```python
from build123d import *

# Parameters (mm, degrees)
SKETCH1_W            = 63
SKETCH1_H            = 76
BOSS_EXTRUDE1_DEPTH  = 1.5
SKETCH2_W            = 9
SKETCH2_H            = 74
BOSS_EXTRUDE2_DEPTH  = 11.5
SKETCH3_W            = 7
SKETCH3_H            = 8
BOSS_EXTRUDE3_DEPTH  = 3.5
SKETCH4_W            = 11
SKETCH4_H            = 2
BOSS_EXTRUDE4_DEPTH  = 3
SKETCH5_R            = 0.325
BOSS_EXTRUDE5_DEPTH  = 6
SKETCH6_W            = 6
SKETCH6_H            = 2
BOSS_EXTRUDE6_DEPTH  = 2.5
SKETCH8_W            = 7.2
SKETCH8_H            = 5.5
BOSS_EXTRUDE8_DEPTH  = 4.2
SKETCH9_W            = 5.5
SKETCH9_H            = 6.1
BOSS_EXTRUDE9_DEPTH  = 2
SKETCH10_R           = 1.5
BOSS_EXTRUDE10_DEPTH = 1.7
SKETCH11_W           = 5.5
SKETCH11_H           = 6.1
BOSS_EXTRUDE11_DEPTH = 2
SKETCH12_R           = 1.5
BOSS_EXTRUDE12_DEPTH = 1.7


with BuildPart() as part:
    # Sketch1 → Boss-Extrude1 (new body)
    with BuildSketch(Plane(origin=(0, 0, 0), x_dir=(1, 0, 0), z_dir=(0, 1, 0))):
        with Locations((31.5, 38)):
            Rectangle(SKETCH1_W, SKETCH1_H)
    extrude(amount=BOSS_EXTRUDE1_DEPTH)

    # Sketch2 → Boss-Extrude2 (add)
    with BuildSketch(Plane(origin=(0, 1.5, 0), x_dir=(1, 0, 0), z_dir=(0, 1, 0))):
        with Locations((7, 38)):
            Rectangle(SKETCH2_W, SKETCH2_H)
    extrude(amount=BOSS_EXTRUDE2_DEPTH)

    # Sketch3 → Boss-Extrude3 (add)
    with BuildSketch(Plane.XZ):
        with Locations((12.5, -19)):
            Rectangle(SKETCH3_W, SKETCH3_H)
        with Locations((12.5, -38)):
            Rectangle(SKETCH3_W, SKETCH3_H)
        with Locations((12.5, -60)):
            Rectangle(SKETCH3_W, SKETCH3_H)
    extrude(amount=BOSS_EXTRUDE3_DEPTH)

    # Sketch4 → Boss-Extrude4 (add)
    with BuildSketch(Plane(origin=(0, 1.5, 0), x_dir=(1, 0, 0), z_dir=(0, 1, 0))):
        with Locations((32.9, 72.5)):
            Rectangle(SKETCH4_W, SKETCH4_H)
    extrude(amount=BOSS_EXTRUDE4_DEPTH)

    # Sketch5 → Boss-Extrude5 (add)
    with BuildSketch(Plane(origin=(0, 4.5, 0), x_dir=(1, 0, 0), z_dir=(0, 1, 0))):
        with Locations((28.6, 72.5)):
            Circle(SKETCH5_R)
        with Locations((31.46, 72.5)):
            Circle(SKETCH5_R)
        with Locations((34.32, 72.5)):
            Circle(SKETCH5_R)
        with Locations((37.18, 72.5)):
            Circle(SKETCH5_R)
    extrude(amount=BOSS_EXTRUDE5_DEPTH)

    # Sketch6 → Boss-Extrude6 (add)
    with BuildSketch(Plane(origin=(0, 1.5, 0), x_dir=(1, 0, 0), z_dir=(0, 1, 0))):
        with Locations((59, 61)):
            Rectangle(SKETCH6_W, SKETCH6_H)
    extrude(amount=BOSS_EXTRUDE6_DEPTH)

    # Sketch8 → Boss-Extrude8 (add)
    with BuildSketch(Plane(origin=(0, 1.5, 0), x_dir=(1, 0, 0), z_dir=(0, 1, 0))):
        with Locations((40.7, 29.25)):
            Rectangle(SKETCH8_W, SKETCH8_H)
        with Locations((49.4, 29.25)):
            Rectangle(SKETCH8_W, SKETCH8_H)
        with Locations((40.7, 20.45)):
            Rectangle(SKETCH8_W, SKETCH8_H)
    extrude(amount=BOSS_EXTRUDE8_DEPTH)

    # Sketch9 → Boss-Extrude9 (add)
    with BuildSketch(Plane(origin=(0, 1.5, 0), x_dir=(1, 0, 0), z_dir=(0, 1, 0))):
        with Locations((59.55, 20.95)):
            Rectangle(SKETCH9_W, SKETCH9_H)
    extrude(amount=BOSS_EXTRUDE9_DEPTH)

    # Sketch10 → Boss-Extrude10 (add)
    with BuildSketch(Plane(origin=(0, 3.5, 0), x_dir=(1, 0, 0), z_dir=(0, 1, 0))):
        with Locations((59.55, 20.95)):
            Circle(SKETCH10_R)
    extrude(amount=BOSS_EXTRUDE10_DEPTH)

    # Sketch11 → Boss-Extrude11 (add)
    with BuildSketch(Plane(origin=(0, 1.5, 0), x_dir=(1, 0, 0), z_dir=(0, 1, 0))):
        with Locations((50.75, 7.95)):
            Rectangle(SKETCH11_W, SKETCH11_H)
    extrude(amount=BOSS_EXTRUDE11_DEPTH)

    # Sketch12 → Boss-Extrude12 (add)
    with BuildSketch(Plane(origin=(0, 3.5, 0), x_dir=(1, 0, 0), z_dir=(0, 1, 0))):
        with Locations((50.75, 7.95)):
            Circle(SKETCH12_R)
    extrude(amount=BOSS_EXTRUDE12_DEPTH)


solid = part.part
```
Here's how the part is built. I have some questions about the finished solid (model axes, mm). A direction names the side the tool comes from. Give positions to 0.01 mm unless a question says otherwise; leave off trailing zeros. Order: outer loops, then holes, each group sorted by start corner. A loop starts at its lowest first (then second) coordinate and runs counter-clockwise, first axis right, second up. Notation, with made-up numbers: (59, 88) -> (106, 88) arc R12 cw to (106, 109) -> close; hole circle Ø4 at (52.5, 0). An arc over 180 degrees is marked (long way). Use CSV: the item, a comma, the result in double quotes. Start each with the question number.
Item 1: If I drill on probe 1 along X at (y, z) = (8, -72.5) (3 decimals); probe 2 along Z at (x, y) = (59, 2.25); probe 3 along X at (y, z) = (4, -18.5), over which ranges is the centre line in solid material (lowest first)? Write a range as [from, to].
Item 2: Suppose I cut it at A-A (y = -1). List the corners of the cut face in (x, z) for me, and give its area (3 significant figures).
Item 3: I'm going to push flat-ended pins straight in: P1, Ø1, axis at x = 20.5, z = -35, coming from the +Y side; P2, Ø1.3, axis at y = 4.5, z = -20, coming from the -X side; P3, Ø1.2, axis at x = 60, y = 3, coming from the -Z side; P4, Ø1.5, axis at y = 1, z = -53.5, coming from the -X side. Where does each tip first touch, or does it pass through?
Item 4: Suppose I cut it at D-D (z = -7.95). List the corners of the cut face in (x, y) for me.
Item 5: Suppose I cut it at C-C (z = -57.5). List the corners of the cut face in (x, y) for me, and give its area (4 significant figures).
Item 6: Suppose I cut it at B-B (x = 59.55). List the corners of the cut face in (y, z) for me, and give its area (3 significant figures).
Item 7: On a 3-axis mill with a long thin cutter (end or side, diameter ignored), from which of +Z, -Z, +X, -X, +Y, -Y can I reach the whole of each face in a straight line? I mean faces 4 (the flat face through (7, 7, -1)), 5 (the flat face through (48, 2, -8)), 6 (the flat face through (56, 3, -61)). Say none if no direction works.
Item 8: Thinking about a two-plate mould opening in Z: for faces 1 (the flat face through (12, -2, -15)), 2 (the flat face through (38.4, 3, -72)), 3 (the flat face through (59, 3, -60)), which applies, pulls with the +Z half, pulls with the -Z half, needs draft (parallel to the pull), parting line crosses it, or undercut?
Answer block:
1,probe 1,"x = [2.5, 11.5], [28.275, 28.925], [31.135, 31.785], [33.995, 34.645], [36.855, 37.505]"
1,probe 2,"z = [-62, -60], [-24, -17.9]"
1,probe 3,"x = [2.5, 11.5], [37.1, 44.3]"
2,outline,"(9, -64) -> (16, -64) -> (16, -56) -> (9, -56) -> close; (9, -42) -> (16, -42) -> (16, -34) -> (9, -34) -> close; (9, -23) -> (16, -23) -> (16, -15) -> (9, -15) -> close"
2,area,"168 mm^2"
3,P1,"stops at y = 1.5"
3,P2,"stops at x = 2.5"
3,P3,"stops at z = -62"
3,P4,"stops at x = 0"
4,outline,"(0, 0) -> (63, 0) -> (63, 1.5) -> (53.5, 1.5) -> (53.5, 3.5) -> (52.25, 3.5) -> (52.25, 5.2) -> (49.25, 5.2) -> (49.25, 3.5) -> (48, 3.5) -> (48, 1.5) -> (11.5, 1.5) -> (11.5, 13) -> (2.5, 13) -> (2.5, 1.5) -> (0, 1.5) -> close"
5,outline,"(0, 0) -> (9, 0) -> (9, -3.5) -> (16, -3.5) -> (16, 0) -> (63, 0) -> (63, 1.5) -> (11.5, 1.5) -> (11.5, 13) -> (2.5, 13) -> (2.5, 1.5) -> (0, 1.5) -> close"
5,area,"222.5 mm^2"
6,outline,"(0, -76) -> (1.5, -76) -> (1.5, -62) -> (4, -62) -> (4, -60) -> (1.5, -60) -> (1.5, -24) -> (3.5, -24) -> (3.5, -22.45) -> (5.2, -22.45) -> (5.2, -19.45) -> (3.5, -19.45) -> (3.5, -17.9) -> (1.5, -17.9) -> (1.5, 0) -> (0, 0) -> close"
6,area,"136 mm^2"
7,face 4,"+Z, +X, -X, +Y"
7,face 5,"+Z, +Y"
7,face 6,"+Z, -Z, +Y"
8,face 1,"pulls with the +Z half"
8,face 2,"needs draft"
8,face 3,"undercut"
